Autodesk Inventor part; units mm, degrees
ref_plane "YZ Plane" through (0, 0, 0) normal (1, 0, 0) x (0, 1, 0)
ref_plane "XZ Plane" through (0, 0, 0) normal (0, 1, 0) x (-1, 0, 0)
ref_plane "XY Plane" through (0, 0, 0) normal (0, 0, 1) x (1, 0, 0)
sketch "Szkic1" plane through (0, 0, 0) normal (0, 1, 0) x (-1, 0, 0)
  circle A0 centre (0, 0) radius 4.25
  line L0 (1.1547, 2) -> (2.3094, 0)
  line L1 (2.3094, 0) -> (1.1547, -2)
  line L2 (1.1547, -2) -> (-1.1547, -2)
  line L3 (-1.1547, -2) -> (-2.3094, 0)
  line L4 (-2.3094, 0) -> (-1.1547, 2)
  line L5 (-1.1547, 2) -> (1.1547, 2)
  circle A1 centre (0, 0) radius 2.5
  dimension "d0" = 8.5
  dimension "d1" = 4
  dimension "d2" = 5
extrude "Wyciągnięcie proste1" add sketch "Szkic1" along normal blind 2 contours A0 | L0 L1 L2 L3 L4 L5 | A1
extrude "Wyciągnięcie proste2" add sketch "Szkic1" against normal blind 3 contours A0 | A1
sketch "Szkic2" plane through (0, 2, 0) normal (0, 1, 0) x (1, 0, 0)
  circle A0 centre (0, 0) radius 2.5
  dimension "d7" = 5
extrude "Wyciągnięcie proste3" add sketch "Szkic2" along normal blind 65
thread "Gwint1"
properties part number "M5x65" material "Aluminum 6061"
Here's how the part is built. I have some questions about the finished solid (model axes, mm). A direction names the side the tool comes from. Round coordinates to 2 decimals unless told otherwise and drop trailing zeros. Loops run counter-clockwise (first coordinate to the right, second up) from the corner with the lowest first, then second, coordinate; pieces in that order, holes last. Notation, with made-up numbers: (59, 46.5) -> (85, 46.5) arc R26 ccw to (85, 72.5) -> close; hole circle Ø4 at (37, -16.75). An arc over 180 degrees is marked (long way). Answer as CSV lines item,"result". Start each with the question number.
1. I need wall thicknesses on probe 1 along Y at (x, z) = (2, 2); probe 2 along Z at (x, y) = (-1.5, 21.5); probe 3 along Y at (x, z) = (0.25, 1.75). Which ranges of each line are inside material? Lowest first, please. Write a range as from..to.
2. For faces 1 (the face through (0, -1, -2)), 2 (the face through (0, 67, 0)), 3 (the face through (-2, 2, -2)), which set-ups out of +Z, -Z, +X, -X, +Y, -Y let a thin tool reach every point of the face, with its end or its side?
3. Imagine slicing it at B-B on z = 0.75. Write out the boundary of the cut face in (x, y).
4. I'm going to push flat-ended pins straight in: P1, Ø1.2, axis at x = 1, z = 0.5, coming from the -Y side; P2, Ø4, axis at x = -1, y = 9, coming from the -Z side; P3, Ø1.2, axis at x = -0.5, y = -2, coming from the -Z side; P4, Ø2, axis at y = 13, z = 2, coming from the -X side. Where does each tip first touch, or does it pass through?
5. Imagine slicing it at C-C on y = 39.5. Write out the boundary of the cut face in (x, z), plus the area to 3 significant figures.
6. Imagine slicing it at A-A on x = 0. Write out the boundary of the cut face in (y, z).
7. If we mould it in two halves opening along Z, with no side actions, what happens to faces 4 (the face through (-2.285, -0.535, -3.584)), 5 (the face through (-1.74, -1.48, -0.99)), 6 (the face through (-2, -3, -1))? For each: pulls with the +Z half, pulls with the -Z half, needs draft (parallel to the pull), parting line crosses it, or undercut.
8. Imagine slicing it at D-D on z = -3.5. Write out the boundary of the cut face in (x, y).
Solution:
1,probe 1,"-3..2"
1,probe 2,"-2..2"
1,probe 3,"0..67"
2,face 1,"-Y"
2,face 2,"+Z, -Z, +X, -X, +Y"
2,face 3,"+Y"
3,outline,"(-4.18, -3) -> (-1.88, -3) -> (-1.88, 0) -> (1.88, 0) -> (1.88, -3) -> (4.18, -3) -> (4.18, 2) -> (2.38, 2) -> (2.38, 67) -> (-2.38, 67) -> (-2.38, 2) -> (-4.18, 2) -> close"
4,P1,"y = 0"
4,P2,"z = -2.5"
4,P3,"z = -4.25"
4,P4,"x = -2.29"
5,outline,"circle Ø5 at (0, 0)"
5,area,"19.6 mm²"
6,outline,"(-3, -4.25) -> (2, -4.25) -> (2, -2.5) -> (67, -2.5) -> (67, 2.5) -> (2, 2.5) -> (2, 4.25) -> (-3, 4.25) -> (-3, 2) -> (0, 2) -> (0, -2) -> (-3, -2) -> close"
7,face 4,"parting line crosses it"
7,face 5,"undercut"
7,face 6,"needs draft"
8,outline,"(-2.41, -3) -> (2.41, -3) -> (2.41, 2) -> (-2.41, 2) -> close"
